from build123d import *

# Parameters (mm, degrees)
SKETCH1_W                               = 180
SKETCH1_H                               = 169
BOSS_EXTRUDE1_DEPTH                     = 14
F_6_0_6_DIAMETER_HOLE1_D                = 6
F_6_0_6_DIAMETER_HOLE1_DEPTH            = 10
M48_CLEARANCE_HOLE1_D                   = 56
M48_CLEARANCE_HOLE1_DEPTH               = 4
F_3_3_3_3_DIAMETER_HOLE1_D              = 3.3
F_3_3_3_3_DIAMETER_HOLE1_DEPTH          = 8
CBORE_FOR_M8_HEX_HEAD_BOLT1_D           = 9
CBORE_FOR_M8_HEX_HEAD_BOLT1_CBORE_D     = 15
CBORE_FOR_M8_HEX_HEAD_BOLT1_CBORE_DEPTH = 8
F_3_3_3_3_DIAMETER_HOLE2_D              = 3.3
F_3_3_3_3_DIAMETER_HOLE2_DEPTH          = 10


with BuildPart() as part:
    # Sketch1 → Boss-Extrude1 (new body)
    with BuildSketch(Plane.XY.offset(14)):
        with Locations((0, 5.5)):
            Rectangle(SKETCH1_W, SKETCH1_H)
    extrude(amount=-BOSS_EXTRUDE1_DEPTH)

    # Ø6.0 (6) Diameter Hole1
    with Locations(Plane.XY.offset(14)):
        with Locations((55, -40), (-55, -40)):
            Hole(F_6_0_6_DIAMETER_HOLE1_D / 2, depth=F_6_0_6_DIAMETER_HOLE1_DEPTH)

    # M48 Clearance Hole1
    with Locations(Plane.XY.offset(14)):
        with Locations((0, 0)):
            Hole(M48_CLEARANCE_HOLE1_D / 2, depth=M48_CLEARANCE_HOLE1_DEPTH)

    # Ø3.3 (3.3) Diameter Hole1
    with Locations(Plane.XY.offset(14)):
        with Locations((23, 31.25), (-11.64, 31.25)):
            Hole(F_3_3_3_3_DIAMETER_HOLE1_D / 2, depth=F_3_3_3_3_DIAMETER_HOLE1_DEPTH)

    # CBORE for M8 Hex Head Bolt1 (through all)
    with Locations(Plane.XY.offset(14)):
        with Locations((40.316, 30.077), (-39.684, 30.077), (40.316, -49.923), (-39.684, -49.923)):
            CounterBoreHole(CBORE_FOR_M8_HEX_HEAD_BOLT1_D / 2, CBORE_FOR_M8_HEX_HEAD_BOLT1_CBORE_D / 2, CBORE_FOR_M8_HEX_HEAD_BOLT1_CBORE_DEPTH)

    # Ø3.3 (3.3) Diameter Hole2
    with Locations(Plane(origin=(0, 90, 0), x_dir=(1, 0, 0), z_dir=(0, 1, 0))):
        with Locations((-12.5, -7), (12.5, -7)):
            Hole(F_3_3_3_3_DIAMETER_HOLE2_D / 2, depth=F_3_3_3_3_DIAMETER_HOLE2_DEPTH)


solid = part.part
Verification items for the finished model (mm, model axes). A direction names the side the tool comes from. Round coordinates to 2 decimals unless told otherwise and drop trailing zeros. Loops run counter-clockwise (first coordinate to the right, second up) from the corner with the lowest first, then second, coordinate; pieces in that order, holes last. Notation, with made-up numbers: (32.5, 62) - (55.5, 62) arc R20 cw to (55.5, 73) - close; hole circle Ø8 at (82, 40). An arc over 180 degrees is marked (long way). Write item = value, one per line.
Q1. Sectioned sample at C-C on y = 0. Record the boundary of the cut face in (x, z).
Here are the results:
outline = (-90, 0) - (90, 0) - (90, 14) - (28, 14) - (28, 10) - (-28, 10) - (-28, 14) - (-90, 14) - close
Q2. Sectioned sample at A-A on y = -40. Record the boundary of the cut face in (x, z), plus the area to 3 significant figures.
Here are the results:
outline = (-90, 0) - (90, 0) - (90, 14) - (58, 14) - (58, 4) - (52, 4) - (52, 14) - (-52, 14) - (-52, 4) - (-58, 4) - (-58, 14) - (-90, 14) - close
area = 2,400 mm^2
Q3. Material ranges on L1, parallel to X at y = -40.5, z = 6.75; L2, parallel to Z at x = -13, y = -10.5; L3, parallel to X at y = -21.5, z = 13, recorded low to high.
Here are the results:
L1 = -90 to -57.96, -52.04 to 52.04, 57.96 to 90
L2 = 0 to 10
L3 = -90 to -17.94, 17.94 to 90
Q4. Sectioned sample at B-B on z = 12. State how many separate pieces and enclosed holes the cut face has, plus the area to 3 significant figures.
Here are the results:
separate_pieces = 1
enclosed_holes = 9
area = 27,200 mm^2
Q5. Mould release check, pull along X, two halves, no side actions. Record for faces 3 (the flat face through (0, 0, 10)), 4 (the flat face through (90, 4, 7)), 5 (the flat face through (19, 25, 14)): +X half, -X half, draft (parallel to the pull), parting line (faces both ways), or undercut.
Here are the results:
face_3 = undercut
face_4 = +X half
face_5 = draft
Q6. Depth check by flat-ended pin: pin 1 (3 mm diameter, centred on x = 23, y = 31.25, fed in from +Z); pin 2 (1.8 mm diameter, centred on x = 56, y = -41, fed in from +Z). Enter the tip coordinate at first touch or a pass-through.
Here are the results:
pin_1 = 6
pin_2 = 4
Q7. Tool access check on faces 1 (the cylindrical face through (47.47, 32.33, 10.06)), 2 (the cylindrical face through (-43.976, 31.429, 2.958)). Record the directions out of +Z, -Z, +X, -X, +Y, -Y that give a thin tool (end or side, any length) a straight path to the whole face; none if there is none.
Here are the results:
face_1 = +Z
face_2 = +Z, -Z
